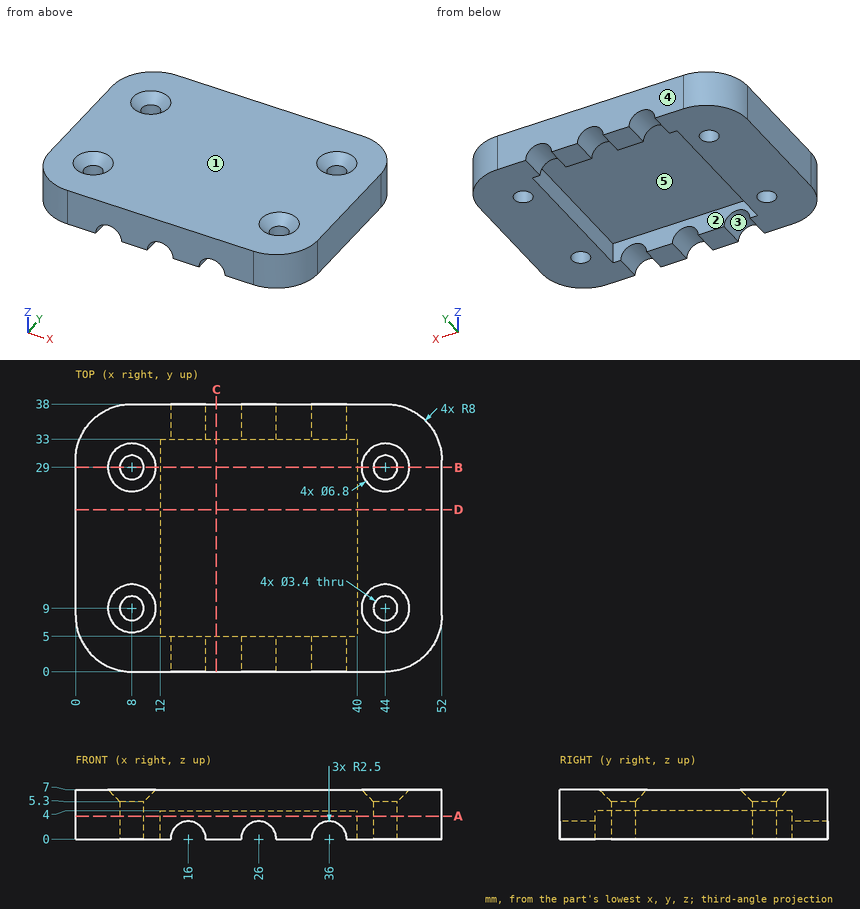
Part print with two shaded views. Sizes in mm from the minimum x, y, z corner. A direction names the side the tool comes from. Give positions to 0.01 mm unless a question says otherwise; leave off trailing zeros. Order: outer loops, then holes, each group sorted by start corner. A loop starts at its lowest first (then second) coordinate and runs counter-clockwise, first axis right, second up.
1) Saw through at C-C, the plane x = 20. Write the cut outline in (y, z), then the cut area to 3 significant figures.
2) Pin check, flat tips, straight feed: pin 1 (2 mm diameter, centred on x = 31, y = 28, fed in from -Z); pin 2 (5.5 mm diameter, centred on x = 44, y = 9, fed in from +Z). Stop position of each tip, or through.
3) Saw through at D-D, the plane y = 23. Write the cut outline in (x, z).
4) Saw through at A-A, the plane z = 3.25. Write the cut outline in (x, y), then the cut area to 3 significant figures.
5) Saw through at B-B, the plane y = 29. Write the cut outline in (x, z).
6) Wall check: probe 1 along Y at (x, z) = (8, 3.45); probe 2 along X at (y, z) = (10.5, 0.5); probe 3 along Z at (x, y) = (28, 15.5). Give the ranges that are in metal, low to high.
7) 3-axis set-ups, long thin cutter, end or side, ignore diameter. For the marked faces 1 and 2: which of +Z, -Z, +X, -X, +Y, -Y reach the whole face in a straight line?
8) Mould opens along Y. For the marked faces 3, 4 and 5 say: +Y half, -Y half, draft (parallel to the pull), parting line (faces both ways), or undercut.
Computed:
1. outline: (0, 0) - (5, 0) - (5, 4) - (33, 4) - (33, 0) - (38, 0) - (38, 7) - (0, 7) - close
1. area: 154 mm2
2. pin 1: stops at z = 4
2. pin 2: stops at z = 6.35
3. outline: (0, 0) - (12, 0) - (12, 4) - (40, 4) - (40, 0) - (52, 0) - (52, 7) - (0, 7) - close
4. outline: (0, 8) arc R8 ccw to (8, 0) - (44, 0) arc R8 ccw to (52, 8) - (52, 30) arc R8 ccw to (44, 38) - (8, 38) arc R8 ccw to (0, 30) - close; hole circle Ø3.4 at (8, 9); hole circle Ø3.4 at (8, 29); hole (12, 5) - (40, 5) - (40, 33) - (12, 33) - close; hole circle Ø3.4 at (44, 9); hole circle Ø3.4 at (44, 29)
4. area: 1,100 mm2
5. outline: (0, 0) - (6.3, 0) - (6.3, 5.3) - (4.6, 7) - (0, 7) - close; (9.7, 0) - (12, 0) - (12, 4) - (40, 4) - (40, 0) - (42.3, 0) - (42.3, 5.3) - (40.6, 7) - (11.4, 7) - (9.7, 5.3) - close; (45.7, 0) - (52, 0) - (52, 7) - (47.4, 7) - (45.7, 5.3) - close
6. probe 1: y = 0 to 7.3, 10.7 to 27.3, 30.7 to 38
6. probe 2: x = 0 to 7.2, 8.8 to 12, 40 to 43.2, 44.8 to 52
6. probe 3: z = 4 to 7
7. face 1: +Z, +X, -X, +Y, -Y
7. face 2: -Z
8. face 3: draft
8. face 4: +Y half
8. face 5: undercut
